CAD build for the part. Positions are in the model's coordinates, mm. Face numbers are marked on the shaded views. A direction names the side the tool comes from. Give positions to 0.01 mm unless a question says otherwise; leave off trailing zeros. Write each loop counter-clockwise with the first axis right and the second up, starting at its lowest first coordinate (ties: lowest second). Pieces come first, ordered by that corner, then holes. Notation, with made-up numbers: (25, 14) - (39, 14) arc R29 ccw to (39, 51) - close; hole circle Ø2 at (27.25, -11). An arc over 180 degrees is marked (long way). Answer as a JSON object with one key per item and string values.
from build123d import *

# Parameters (mm, degrees)
F0_W     = 50.8
F0_H     = 6.35
F1_DEPTH = 19.05
F2_W     = 12.065
F2_H     = 19.05
F3_DEPTH = 20.32
F4_SIZE2 = 10.16
F4_SIZE  = 20.32
F5_SIZE2 = 20.31999
F5_SIZE  = 10.15999


# Not quite as in the source:
# - a fillet or chamfer is up to 0.001 mm smaller than in the source, because OpenCascade refuses the exact size


with BuildPart() as f1:
    # F0 (on Front) → F1 (new body)
    with BuildSketch(Plane.XZ):
        with Locations((25.4, -3.175)):
            Rectangle(F0_W, F0_H)
    extrude(amount=F1_DEPTH)

    # F2 (on face) → F3 (join)
    with BuildSketch(Plane.XY):
        with Locations((44.7675, -9.525)):
            Rectangle(F2_W, F2_H)
    extrude(amount=F3_DEPTH)

    # F4
    f4_edges = [f1.edges().sort_by_distance(p)[0] for p in [
        (50.8, -9.525, -6.35),
    ]]
    f4_side = f1.faces().sort_by_distance((50.8, -9.525, 6.985))[0]
    chamfer(f4_edges, length=F4_SIZE, length2=F4_SIZE2, reference=f4_side)

    # F5 (size 10.16 and 20.32 in the source; OpenCascade refuses exactly that, so slightly less here)
    f5_edges = [f1.edges().sort_by_distance(p)[0] for p in [
        (38.735, -9.525, 20.32),
    ]]
    f5_side = f1.faces().sort_by_distance((44.7675, -9.525, 20.32))[0]
    chamfer(f5_edges, length=F5_SIZE, length2=F5_SIZE2, reference=f5_side)


solid = f1.part
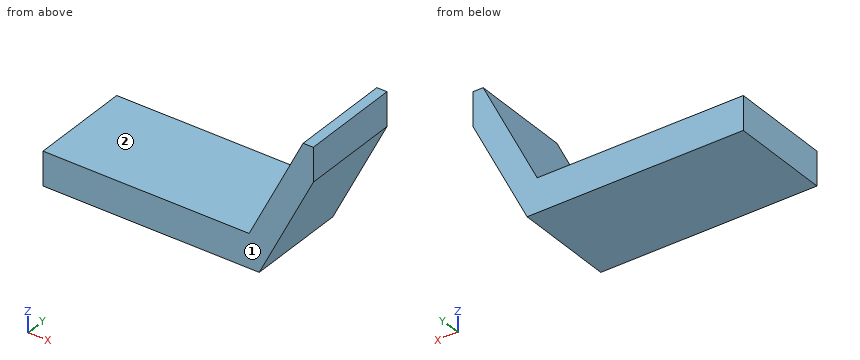
(1) 3-axis set-ups, long thin cutter, end or side, ignore diameter. For the marked faces 1 and 2: which of +Z, -Z, +X, -X, +Y, -Y reach the whole face in a straight line?
Answer key:
{"face 1": "+Z, -Z, +X, -X, -Y", "face 2": "+Z, -X, +Y, -Y"}
(2) Saw through at C-C, the plane z = 18.75. Give the cut face in (x, y).
Answer key:
{"outline": "(48.11, -19.05) - (50.8, -19.05) - (50.8, 0) - (48.11, 0) - close"}
(3) Saw through at B-B, the plane x = 6. Give the cut face in (y, z), and give its area (3 significant figures).
Answer key:
{"outline": "(-19.05, -6.35) - (0, -6.35) - (0, 0) - (-19.05, 0) - close", "area": "121 mm²"}
(4) Probe L1, parallel to Z at x = 29.5, y = -12; L2, parallel to X at y = -11.25, z = 8.5 (3 decimals). List the from-to ranges inside material, lowest first. Write a range as [from, to].
Answer key:
{"L1": "z = [-6.35, 0]", "L2": "x = [42.985, 48.065]"}
(5) Flat gauge pins, fed straight in: P1, Ø1, axis at x = 16, y = -5.5, coming from the +Z side; P2, Ø10, axis at x = 5.5, z = 0, coming from the +Y side; P3, Ø8, axis at y = -9.5, z = 7, coming from the +X side (3 decimals); P4, Ø1.5, axis at y = -8.5, z = 4, coming from the -X side. Where does each tip first touch, or does it go through?
Answer key:
{"P1": "stops at z = 0", "P2": "stops at y = 0", "P3": "stops at x = 49.315", "P4": "stops at x = 40.36"}
